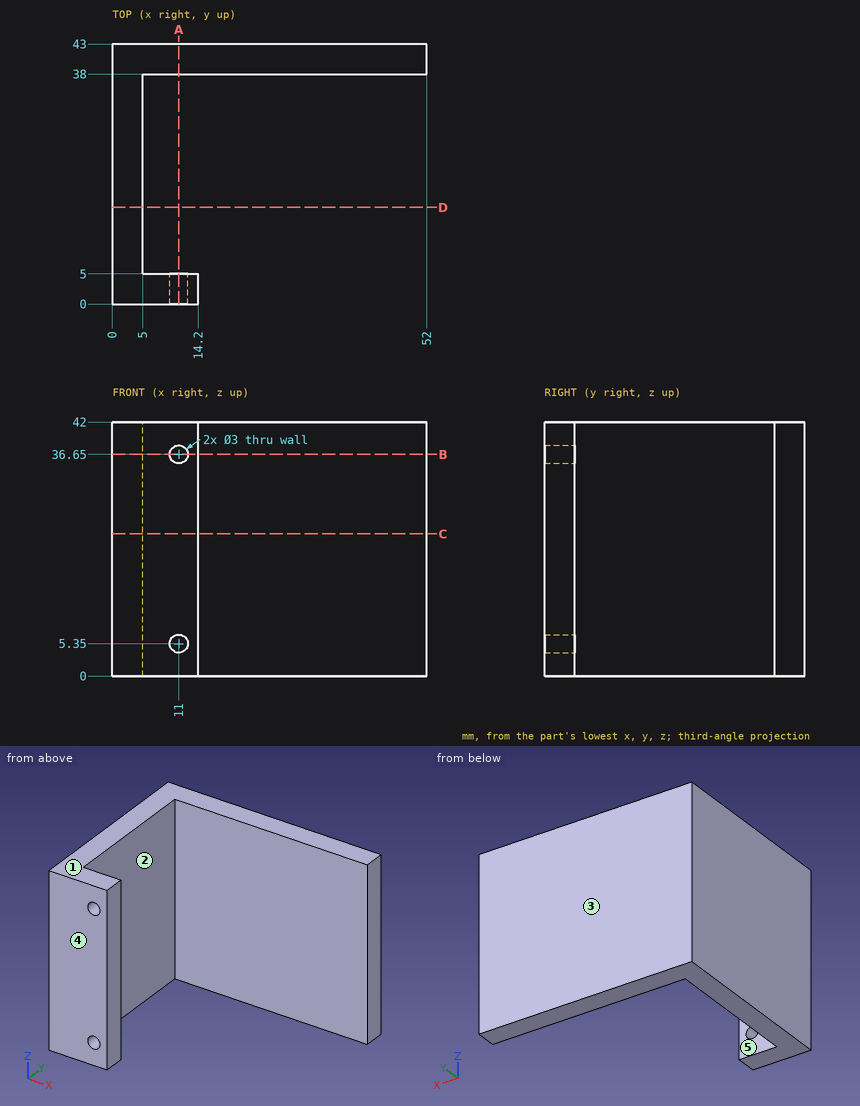
Design review of the part shown in the three views and the two pictorial views. Dimensions are in mm from the part's minimum x, y and z. A direction names the side the tool comes from. Round coordinates to 2 decimals unless told otherwise and drop trailing zeros. Write each loop counter-clockwise with the first axis right and the second up, starting at its lowest first coordinate (ties: lowest second). Pieces come first, ordered by that corner, then holes. Notation, with made-up numbers: (-12.5, 84) - (5.5, 84) arc R14 cw to (5.5, 92) - close; hole circle Ø1 at (65.25, 77.25). An arc over 180 degrees is marked (long way). Write item = value, one per line. Start each with the question number.
1. Consider section A-A on x = 11. State the section outline as (y, z) points.
2. For the marked faces 1 and 2, list the 3-axis set-ups (+Z, -Z, +X, -X, +Y, -Y) from which the entire face can be reached by the end or side of a thin tool; tool diameter is ignored.
3. Wall thickness on L1, parallel to Z at x = 11, y = 2.65; L2, parallel to Y at x = 9.5, z = 23.5; L3, parallel to Y at x = 46, z = 30: over which ranges is each line inside the solid? List them lowest first.
4. For pin 1 Ø2 at (x, z) = (16.5, 6) entering from -Y; pin 2 Ø3 at (y, z) = (12, 35) entering from +X; pin 3 Ø5.5 at (y, z) = (3.5, 28.5) entering from +X, all flat-tipped, find the tip position at first contact; note any pin that passes through.
5. Consider section B-B on z = 36.65. State the section outline as (x, y) points.
6. Draft analysis for pull direction Y (two halves, no side actions). For the marked faces 3, 4 and 5, state which applies: released by +Y, released by -Y, zero draft, split by the parting line, or undercut.
7. Consider section D-D on y = 16. State the section outline as (x, z) points, plus the area to 3 significant figures.
8. Consider section C-C on z = 23.5. State the section outline as (x, y) points.
Evaluation:
q1.outline = (0, 0) - (5, 0) - (5, 3.85) - (0, 3.85) - close; (0, 6.85) - (5, 6.85) - (5, 35.15) - (0, 35.15) - close; (0, 38.15) - (5, 38.15) - (5, 42) - (0, 42) - close; (38, 0) - (43, 0) - (43, 42) - (38, 42) - close
q2.face_1 = +Z, +X, -X, +Y, -Y
q2.face_2 = +Z, -Z, +X
q3.L1 = 0 to 3.85, 6.85 to 35.15, 38.15 to 42
q3.L2 = 0 to 5, 38 to 43
q3.L3 = 38 to 43
q4.pin_1 = 38
q4.pin_2 = 5
q4.pin_3 = 14.2
q5.outline = (0, 0) - (9.5, 0) - (9.5, 5) - (5, 5) - (5, 38) - (52, 38) - (52, 43) - (0, 43) - close; (12.5, 0) - (14.2, 0) - (14.2, 5) - (12.5, 5) - close
q6.face_3 = released by +Y
q6.face_4 = released by -Y
q6.face_5 = undercut
q7.outline = (0, 0) - (5, 0) - (5, 42) - (0, 42) - close
q7.area = 210 mm2
q8.outline = (0, 0) - (14.2, 0) - (14.2, 5) - (5, 5) - (5, 38) - (52, 38) - (52, 43) - (0, 43) - close
